Model file for the job. Use its own axes, mm. Round coordinates to 2 decimals unless told otherwise and drop trailing zeros. Order: outer loops, then holes, each group sorted by start corner. A loop starts at its lowest first (then second) coordinate and runs counter-clockwise, first axis right, second up. Notation, with made-up numbers: (2, 68) - (35, 68) arc R12 ccw to (35, 89) - close; hole circle Ø7 at (21.25, -36). An arc over 180 degrees is marked (long way). Write item = value, one per line. Start each with the question number.
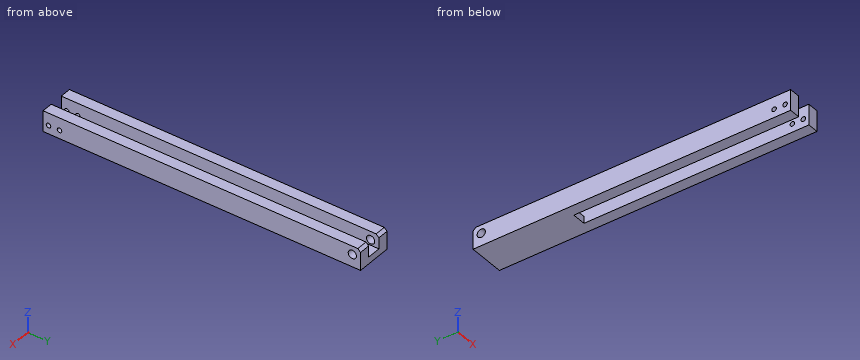
from build123d import *

# Parameters (mm, degrees)
EXTRUDE_1_DEPTH     = 231
SKETCH_2_R          = 3
CUT_EXTRUDE_1_DEPTH = 233.579556281
HOLE_WIZARD_M4_1_D  = 3.3
CHAMFER_1_SIZE      = 2
CUT_EXTRUDE_3_REACH = 233.582
SKETCH_8_W          = 10
SKETCH_8_H          = 168.002742078


with BuildPart() as part:
    # 草图1 → 凸台-拉伸1 (new body)
    with BuildSketch(Plane(origin=(0, 0, 0), x_dir=(1, 0, 0), z_dir=(0, 1, 0))):
        Polygon((-13, -7.5), (-5, -7.5), (-5, 2.5), (5, 2.5), (5, -7.5), (13, -7.5), (13, 7.5), (-13, 7.5), align=None)
    extrude(amount=-EXTRUDE_1_DEPTH)

    # 草图2 → 切除-拉伸1 (cut, through all)
    with BuildSketch(Plane(origin=(13, 0, 0), x_dir=(0, 0, -1), z_dir=(1, 0, 0))):
        with Locations((-1.5, -6)):
            Circle(SKETCH_2_R)
    extrude(amount=-CUT_EXTRUDE_1_DEPTH, mode=Mode.SUBTRACT)

    # M4 螺纹孔1 (through all)
    with Locations(Plane.ZY.offset(13)):
        with Locations((-1.5, -227), (-1.5, -219)):
            Hole(HOLE_WIZARD_M4_1_D / 2)

    # 倒角1
    chamfer_1_edges = [part.edges().sort_by_distance(p)[0] for p in [
        (9, 0, 7.5),
        (-9, 0, 7.5),
    ]]
    chamfer(chamfer_1_edges, length=CHAMFER_1_SIZE)

    # 草图8 → 切除-拉伸3 (cut, up to next)
    with BuildSketch(Plane.XY.offset(-2.5), mode=Mode.PRIVATE) as cut_extrude_3_sk1:
        with Locations((0, -151.451371039)):
            Rectangle(SKETCH_8_W, SKETCH_8_H)
    cut_extrude_3_tool1 = extrude(cut_extrude_3_sk1.sketch, amount=-CUT_EXTRUDE_3_REACH, mode=Mode.PRIVATE) & part.part
    add(cut_extrude_3_tool1.solids().sort_by_distance((0, -151.451371, -2.5))[0], mode=Mode.SUBTRACT)


solid = part.part
Item 1: Saw through at A-A, the plane y = -6. Give the cut face in (x, z).
Item 2: Drop flat-ended pins along their axis: pin 1 (5 mm diameter, centred on x = 1.5, y = -46, fed in from +Z); pin 2 (5.5 mm diameter, centred on x = 1, z = -4.5, fed in from -Y). Give the stop position or say it passes through.
Item 3: Saw through at C-C, the plane x = -2. Give the cut face in (y, z).
Item 4: Saw through at B-B, the plane y = -215. Give the cut face in (x, z).
Item 5: Probe L1, parallel to Z at x = 8, y = -219; L2, parallel to X at y = -180, z = -4.75; L3, parallel to Y at x = 11.25, z = 1.5. List the from-to ranges inside material, lowest first.
Check sheet entries:
q1.outline = (-13, -7.5) - (13, -7.5) - (13, -1.5) - (5, -1.5) - (5, -2.5) - (-5, -2.5) - (-5, -1.5) - (-13, -1.5) - close; (-13, 4.5) - (-5, 4.5) - (-5, 7.5) - (-13, 7.5) - close; (5, 4.5) - (13, 4.5) - (13, 7.5) - (5, 7.5) - close
q2.pin_1 = -2.5
q2.pin_2 = -67.45
q3.outline = (-67.45, -7.5) - (0, -7.5) - (0, -2.5) - (-67.45, -2.5) - close
q4.outline = (-13, -7.5) - (-5, -7.5) - (-5, 7.5) - (-13, 7.5) - close; (5, -7.5) - (13, -7.5) - (13, 7.5) - (5, 7.5) - close
q5.L1 = -7.5 to -3.15, 0.15 to 7.5
q5.L2 = -13 to -5, 5 to 13
q5.L3 = -231 to -9, -3 to 0
